```python
from build123d import *

# Parameters (mm, degrees)
F0_W     = 71.67
F0_H     = 17.78
F1_DEPTH = 8.89
F2_W     = 6
F2_H     = 0.81
F3_DEPTH = 17.781
F4_W     = 58.97
F4_H     = 8.89
F5_DEPTH = 12.7


with BuildPart() as f1:
    # F0 (on Front) → F1 (new body, symmetric)
    with BuildSketch(Plane.XZ):
        Rectangle(F0_W, F0_H)
    extrude(amount=F1_DEPTH, both=True)

    # F2 (on face) → F3 (cut, through all)
    with BuildSketch(Plane.XZ.offset(8.89)):
        with Locations((-22.668, 8.485)):
            Rectangle(F2_W, F2_H)
        with BuildLine():
            Line((-19.668, 8.08), (-25.668, 8.08))
            ThreePointArc((-25.668, 8.08), (-22.668, 5.08), (-19.668, 8.08))
        make_face()
        with Locations((-11.334, 8.485)):
            Rectangle(F2_W, F2_H)
        with BuildLine():
            ThreePointArc((-14.334, 8.08), (-11.334, 5.08), (-8.334, 8.08))
            Line((-8.334, 8.08), (-14.334, 8.08))
        make_face()
        with Locations((0, 8.485)):
            Rectangle(F2_W, F2_H)
        with BuildLine():
            ThreePointArc((-3, 8.08), (0, 5.08), (3, 8.08))
            Line((3, 8.08), (-3, 8.08))
        make_face()
        with Locations((11.334, 8.485)):
            Rectangle(F2_W, F2_H)
        with BuildLine():
            ThreePointArc((8.334, 8.08), (11.334, 5.08), (14.334, 8.08))
            Line((14.334, 8.08), (8.334, 8.08))
        make_face()
        with BuildLine():
            Line((25.668, 8.08), (25.668, 8.89))
            Line((25.668, 8.89), (19.668, 8.89))
            Line((19.668, 8.89), (19.668, 8.08))
            ThreePointArc((19.668, 8.08), (22.668, 5.08), (25.668, 8.08))
        make_face()
    extrude(amount=-F3_DEPTH, mode=Mode.SUBTRACT)

    # F4 (on face) → F5 (cut)
    with BuildSketch(Plane.XZ.offset(8.89)):
        with Locations((0, -4.445)):
            Rectangle(F4_W, F4_H)
    extrude(amount=-F5_DEPTH, mode=Mode.SUBTRACT)


solid = f1.part
```
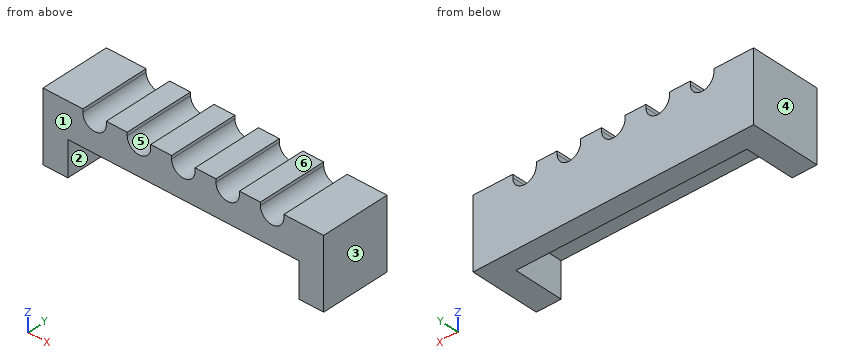
Geometry check sheet. Reference: the model listing, model coordinates, mm. Face numbers are marked on the shaded views. A direction names the side the tool comes from. Give positions to 0.01 mm unless a question says otherwise; leave off trailing zeros. Loops run counter-clockwise (first coordinate to the right, second up) from the corner with the lowest first, then second, coordinate; pieces in that order, holes last. Notation, with made-up numbers: M 84,78 L 139,78 A28 ccw 139,116 Z; hole C 64,64.25 d9. An arc over 180 degrees is marked long. Write item = value, one per line. Start each with the question number.
1. Thickness scan on probe 1 along X at (y, z) = (-6.5, -4.5) (3 decimals); probe 2 along Y at (x, z) = (-11, -4); probe 3 along X at (y, z) = (-2, 7.75) (3 decimals). Record the ranges inside material, lowest first.
2. Tool access check on the marked faces 1 and 2. Record the directions out of +Z, -Z, +X, -X, +Y, -Y that give a thin tool (end or side, any length) a straight path to the whole face; none if there is none.
3. Section check A-A, the plane y = -6.75. Enter the section's corners in (x, z) (3 decimals).
4. Go/stop test with flat-tipped pins: P1, Ø10, axis at x = 6.5, y = -4.5, coming from the -Z side; P2, Ø1, axis at x = 11, y = -4, coming from the +Z side; P3, Ø2.5, axis at x = -5.5, z = -3.5, coming from the -Y side. Record where each tip stops, or that it passes through.
5. Section check D-D, the plane x = 0. Enter the section's corners in (y, z).
6. Section check C-C, the plane z = -2.5. Enter the section's corners in (x, y) (3 decimals), plus the area to 3 significant figures.
7. Draft check along X on the marked faces 3, 4, 5 and 6. Enter one of: +X half, -X half, draft (parallel to the pull), parting line (faces both ways), or undercut.
8. Section check B-B, the plane z = 6.75. Enter the section's corners in (x, y) (3 decimals), plus the area to 3 significant figures.
Values follow:
q1.probe_1 = -35.835 to -29.485, 29.485 to 35.835
q1.probe_2 = 3.81 to 8.89
q1.probe_3 = -35.835 to -25.65, -19.686 to -14.316, -8.352 to -2.982, 2.982 to 8.352, 14.316 to 19.686, 25.65 to 35.835
q2.face_1 = +Z, -Z, +X, -X, -Y
q2.face_2 = -Z, -Y
q3.outline = M -35.835,-8.89 L -29.485,-8.89 L -29.485,0 L 29.485,0 L 29.485,-8.89 L 35.835,-8.89 L 35.835,8.89 L 25.668,8.89 L 25.668,8.08 A3 cw 19.668,8.08 L 19.668,8.89 L 14.334,8.89 L 14.334,8.08 A3 cw 8.334,8.08 L 8.334,8.89 L 3,8.89 L 3,8.08 A3 cw -3,8.08 L -3,8.89 L -8.334,8.89 L -8.334,8.08 A3 cw -14.334,8.08 L -14.334,8.89 L -19.668,8.89 L -19.668,8.08 A3 cw -25.668,8.08 L -25.668,8.89 L -35.835,8.89 Z
q4.P1 = 0
q4.P2 = 5.2
q4.P3 = 3.81
q5.outline = M -8.89,0 L 3.81,0 L 3.81,-8.89 L 8.89,-8.89 L 8.89,5.08 L -8.89,5.08 Z
q6.outline = M -35.835,-8.89 L -29.485,-8.89 L -29.485,3.81 L 29.485,3.81 L 29.485,-8.89 L 35.835,-8.89 L 35.835,8.89 L -35.835,8.89 Z
q6.area = 525 mm^2
q7.face_3 = +X half
q7.face_4 = -X half
q7.face_5 = undercut
q7.face_6 = draft
q8.outline = M -35.835,-8.89 L -25.357,-8.89 L -25.357,8.89 L -35.835,8.89 Z; M -19.979,-8.89 L -14.023,-8.89 L -14.023,8.89 L -19.979,8.89 Z; M -8.645,-8.89 L -2.689,-8.89 L -2.689,8.89 L -8.645,8.89 Z; M 2.689,-8.89 L 8.645,-8.89 L 8.645,8.89 L 2.689,8.89 Z; M 14.023,-8.89 L 19.979,-8.89 L 19.979,8.89 L 14.023,8.89 Z; M 25.357,-8.89 L 35.835,-8.89 L 35.835,8.89 L 25.357,8.89 Z
q8.area = 796 mm^2
